Geometry: final body of the model. Coordinates: model frame, mm. Round coordinates to 2 decimals unless told otherwise and drop trailing zeros. Write each loop counter-clockwise with the first axis right and the second up, starting at its lowest first coordinate (ties: lowest second). Pieces come first, ordered by that corner, then holes. Notation, with made-up numbers: M 75.5,54.5 L 94.5,54.5 A13 cw 94.5,78.5 Z; hole C -14.5,47.5 d5. An arc over 180 degrees is marked long. Answer as CSV lines item,"result". Start each with the question number.
Q1. First-contact query: pin 1 (1.5 mm diameter, centred on x = 3.5, y = -7.5, fed in from +Z); pin 2 (1.5 mm diameter, centred on x = 6.5, y = 8.5, fed in from +Z); pin 3 (3 mm diameter, centred on x = 5.5, y = 4.5, fed in from -Z). Flat tips, straight axial feed; report the tip coordinate or a pass-through.
Q2. Ray query, probe 1 along Z at (x, y) = (6.5, 0); probe 2 along Z at (x, y) = (3.25, 6); probe 3 along Y at (x, z) = (7, -3). Return the intervals inside material, ascending.
Q3. Mould query, pull axis Y, two halves, no side actions, for faces 1 (the cylindrical face through (4.81, -1.72, -7.75)), 2 (the cylindrical face through (2.37, -2.75, 12.4)), 3 (the flat face through (1.588, -0.2, -8.3)). Classes: pulls with the +Y half, pulls with the -Y half, needs draft (parallel to the pull), parting line crosses it, or undercut.
Q4. Section query C-C on x = 2.75. Output: boundary loops of the cut face in (y, z) (1 decimal), and give its area (3 significant figures).
Autodesk Inventor part; units mm, degrees
ref_plane "YZ Plane" through (0, 0, 0) normal (1, 0, 0) x (0, 1, 0)
ref_plane "XZ Plane" through (0, 0, 0) normal (0, 1, 0) x (-1, 0, 0)
ref_plane "XY Plane" through (0, 0, 0) normal (0, 0, 1) x (1, 0, 0)
sketch "Sketch1" plane through (0, 0, 0) normal (0, 0, 1) x (1, 0, 0)
  line L0 (0, 0) -> (9.525, 0) construction
  line L1 (1.5875, 7.9375) -> (7.9375, 7.9375)
  line L2 (7.9375, 7.9375) -> (7.9375, 12.7)
  line L3 (1.5875, 12.7) -> (1.5875, 7.9375)
  line L4 (3.175, 12.7) -> (4.7625, 11.1125)
  line L5 (4.7625, 11.1125) -> (6.35, 12.7)
  line L6 (7.9375, 12.7) -> (6.35, 12.7)
  line L7 (3.175, 12.7) -> (1.5875, 12.7)
  line L8 (1.5875, 7.9375) -> (0, 7.9375)
  line L9 (0, 7.9375) -> (0, 6.6675)
  line L10 (0, 6.6675) -> (0.635, 6.6675)
  line L11 (0.635, 6.6675) -> (0.635, 5.08)
  line L12 (0.635, 5.08) -> (0, 5.08)
  line L13 (0, 5.08) -> (0, 2.54)
  line L14 (0, 2.54) -> (9.525, 2.54)
  line L15 (9.525, 2.54) -> (9.525, 5.08)
  line L16 (9.525, 5.08) -> (8.89, 5.08)
  line L17 (8.89, 5.08) -> (8.89, 6.6675)
  line L18 (8.89, 6.6675) -> (9.525, 6.6675)
  line L19 (9.525, 6.6675) -> (9.525, 7.9375)
  line L20 (9.525, 7.9375) -> (7.9375, 7.9375)
  point P0 (4.7625, 7.9375)
  dimension "d0" = 6.35
  dimension "d1" = 4.7625
  dimension "d2" = 1.5875
  dimension "d3" = 7.9375
  dimension "d5" = 11.1125
  dimension "d6" = 9.525
  dimension "d7" = 1.27
  dimension "d8" = 1.5875
  dimension "d9" = 2.54
  dimension "d10" = 0.635
revolve "Revolution1" add sketch "Sketch1" angle 360 about axis through (0, 0, 0) along (1, 0, 0) contours L3 L7 L4 L5 L6 L2 L1
properties part number "8 ball cable roller"
Entries:
1,pin 1,"stops at z = 10.71"
1,pin 2,"stops at z = 10.06"
1,pin 3,"stops at z = -12.27"
2,probe 1,"z = -12.7 to -7.94, 7.94 to 12.7"
2,probe 2,"z = -11.11 to -5.2, 5.2 to 11.11"
2,probe 3,"y = -12.34 to -7.35, 7.35 to 12.34"
3,face 1,"undercut"
3,face 2,"parting line crosses it"
3,face 3,"needs draft"
4,outline,"C 0,0 d25.4; hole C 0,0 d15.9"
4,area,"309 mm^2"
